```python
from build123d import *

# Parameters (mm, degrees)
F0_W     = 57.15
F0_H     = 63.5
F1_DEPTH = 127
F3_D     = 38.1
F3_DEPTH = 12.7
F3_TIP   = 11.4463947925
F4_R     = 5.08
F6_D     = 3.175


with BuildPart() as f1:
    # F0 (on Top) → F1 (new body)
    with BuildSketch(Plane.XY):
        with Locations((28.575, -31.75)):
            Rectangle(F0_W, F0_H)
    extrude(amount=F1_DEPTH)

    # F3
    with Locations(Plane.XY.offset(127)):
        with Locations((28.575, -31.75)):
            Hole(F3_D / 2, depth=F3_DEPTH)
            with Locations((0, 0, -(F3_DEPTH + F3_TIP / 2))):  # 118° drill point
                Cone(0, F3_D / 2, F3_TIP, mode=Mode.SUBTRACT)

    # F4
    f4_edges = [f1.edges().sort_by_distance(p)[0] for p in [
        (57.15, -31.75, 127),
        (28.575, 0, 127),
        (0, -31.75, 127),
        (28.575, -63.5, 127),
    ]]
    fillet(f4_edges, radius=F4_R)

    # F6 (through all)
    with Locations(Plane(origin=(0, 0, 0), x_dir=(-1, 0, 0), z_dir=(0, 1, 0))):
        with Locations((-28.575, 25.4)):
            Hole(F6_D / 2)


solid = f1.part
```
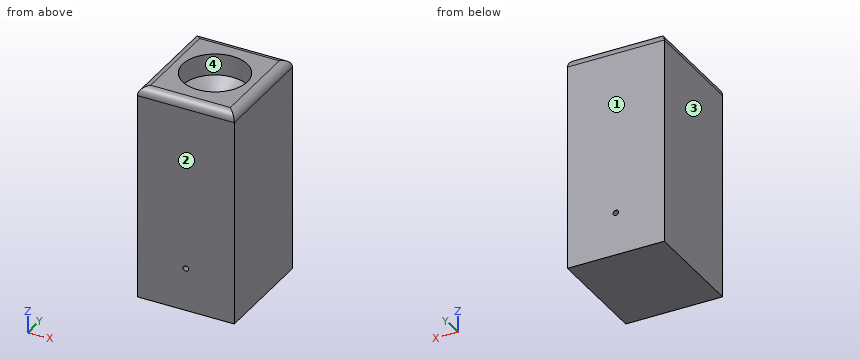
Could you check a few things on this model? Use its own coordinates, in mm. Face numbers are marked on the shaded views. Round coordinates to 2 decimals unless told otherwise and drop trailing zeros. Loops run counter-clockwise (first coordinate to the right, second up) from the corner with the lowest first, then second, coordinate; pieces in that order, holes last. Notation, with made-up numbers: (72, 39.25) -> (98, 39.25) arc R27 ccw to (98, 66.25) -> close; hole circle Ø6 at (85, -39). An arc over 180 degrees is marked (long way). Put each result on its own line as item: value.
Q1. Please list where these lines run through material, in increasing order: line 1 (X direction, y = -31, z = 121); line 2 (Z direction, x = 29, y = -14); line 3 (X direction, y = -32, z = 25). Write a range as from..to.
Checks:
line 1: 0..9.54, 47.61..57.15
line 2: 0..23.87, 26.93..113.52
line 3: 0..27.04, 30.11..57.15
Q2. I want a section at B-B on z = 119. Write out the boundary of the cut face in (x, y) (3 decimals).
Checks:
outline: (0, -63.5) -> (57.15, -63.5) -> (57.15, 0) -> (0, 0) -> close; hole circle Ø38.1 at (28.575, -31.75)
Q3. I want a section at A-A on z = 25.4. Write out the boundary of the cut face in (x, y), and give its area (3 significant figures).
Checks:
outline: (0, -63.5) -> (26.99, -63.5) -> (26.99, 0) -> (0, 0) -> close; (30.16, -63.5) -> (57.15, -63.5) -> (57.15, 0) -> (30.16, 0) -> close
area: 3,430 mm2
Q4. Thinking about a two-plate mould opening in Y: for the marked faces 1, 2, 3 and 4, which applies, pulls with the +Y half, pulls with the -Y half, needs draft (parallel to the pull), parting line crosses it, or undercut?
Checks:
face 1: pulls with the +Y half
face 2: pulls with the -Y half
face 3: needs draft
face 4: undercut
Q5. For pin 1 Ø4 at (x, y) = (30.5, -42) entering from +Z, with a flat end and sliding along its axis, tell me the tip position at first contact or that it passes through.
Checks:
pin 1: z = 110.32
